Autodesk Inventor part; units mm, degrees
ref_plane "BEF_2_XY" through (32, 0, 0) normal (0, 0, 1) x (1, 0, 0)
ref_plane "BEF_2_YZ" through (32, 0, 0) normal (1, 0, 0) x (0, 1, 0)
ref_plane "BEF_2_ZX" through (32, 0, 0) normal (0, 1, 0) x (0, 0, 1)
sketch "Sketch_1" plane through (0, 0, 0) normal (0, 0, 1) x (1, 0, 0)
  line L0 (-12, -22.5) -> (98, -22.5)
  line L1 (98, -22.5) -> (98, 22.5)
  line L2 (98, 22.5) -> (-12, 22.5)
  line L3 (-12, 22.5) -> (-12, -22.5)
extrude "Extrusion1" add sketch "Sketch_1" along normal blind 200
sketch "Sketch_2" plane through (0, 0, 0) normal (0, 1, 0) x (-1, 0, 0)
  line L0 (0, 200) -> (0, 0)
  line L1 (0, 0) -> (-7, 0)
  line L2 (-7, 0) -> (-7, 4)
  line L3 (-7, 4) -> (-5.5, 4)
  line L4 (-5.5, 4) -> (-5.5, 20)
  line L5 (-5.5, 20) -> (-9, 20)
  line L6 (-9, 20) -> (-9, 200)
  line L7 (-9, 200) -> (0, 200)
  line L8 (0, 200) -> (0, 0)
revolve "Revolution1" cut sketch "Sketch_2" angle 360 about axis through (0, 0, 200) along (0, 0, 1)
pattern_linear "Rectangular Pattern1" count 2 spacing 32 along (1, 0, 0) of "Revolution1"
sketch "Sketch_8" plane through (0, 0, 200) normal (0, 0, 1) x (1, 0, 0)
  line L0 (-12, -22.5) -> (37.5, -22.5)
  line L1 (37.5, -22.5) -> (37.5, 22.5)
  line L2 (37.5, 22.5) -> (-12, 22.5)
  line L3 (-12, 22.5) -> (-12, -22.5)
extrude "Extrusion2" cut sketch "Sketch_8" against normal blind 160
sketch "Sketch_17" plane through (0, 22.5, 0) normal (0, 1, 0) x (1, 0, 0)
  arc A0 (37.5, -1.8) -> (37.5, -8.2) centre (37.5, -5) ccw
  line L0 (37.5, -8.2) -> (48.5, -8.2)
  arc A1 (48.5, -8.2) -> (48.5, -1.8) centre (48.5, -5) ccw
  line L1 (48.5, -1.8) -> (37.5, -1.8)
extrude "Extrusion3" cut sketch "Sketch_17" against normal blind 0.75
ref_plane "BEF_2_XY" through (32, 0, 0) normal (0, 0, 1) x (1, 0, 0)
ref_plane "BEF_2_YZ" through (32, 0, 0) normal (1, 0, 0) x (0, 1, 0)
ref_plane "BEF_2_ZX" through (32, 0, 0) normal (0, 1, 0) x (0, 0, 1)
ref_plane "IP_ALU_XY" through (43, 21.75, 5) normal (0, -1, 0) x (1, 0, 0)
ref_plane "IP_ALU_YZ" through (43, 21.75, 5) normal (1, 0, 0) x (0, 0, 1)
ref_plane "IP_ALU_ZX" through (43, 21.75, 5) normal (0, 0, 1) x (0, -1, 0)
ref_plane "IP_ALU_3_7_XY" through (44, 21.75, 5) normal (0, -1, 0) x (1, 0, 0)
ref_plane "IP_ALU_3_7_YZ" through (44, 21.75, 5) normal (1, 0, 0) x (0, 0, 1)
ref_plane "IP_ALU_3_7_ZX" through (44, 21.75, 5) normal (0, 0, 1) x (0, -1, 0)
ref_plane "IP_ALU_5_XY" through (44, 21.75, 5) normal (0, -1, 0) x (1, 0, 0)
ref_plane "IP_ALU_5_YZ" through (44, 21.75, 5) normal (1, 0, 0) x (0, 0, 1)
ref_plane "IP_ALU_5_ZX" through (44, 21.75, 5) normal (0, 0, 1) x (0, -1, 0)
ref_plane "IP_GR_XY" through (0, 0, 0) normal (0, 0, 1) x (1, 0, 0)
ref_plane "IP_GR_YZ" through (0, 0, 0) normal (1, 0, 0) x (0, 1, 0)
ref_plane "IP_GR_ZX" through (0, 0, 0) normal (0, 1, 0) x (0, 0, 1)
ref_plane "IP_SCH_1_XY" through (0, 0, 20) normal (0, 0, 1) x (1, 0, 0)
ref_plane "IP_SCH_1_YZ" through (0, 0, 20) normal (1, 0, 0) x (0, 1, 0)
ref_plane "IP_SCH_1_ZX" through (0, 0, 20) normal (0, 1, 0) x (0, 0, 1)
ref_plane "IP_SCH_2_XY" through (32, 0, 20) normal (0, 0, 1) x (1, 0, 0)
ref_plane "IP_SCH_2_YZ" through (32, 0, 20) normal (1, 0, 0) x (0, 1, 0)
ref_plane "IP_SCH_2_ZX" through (32, 0, 20) normal (0, 1, 0) x (0, 0, 1)
properties part number "FGR AL-2-PGN-plus-P 160,PGN-plus-P 160-2-AS-P81110452001216049.51650000000000000000Aluminium6.5"
Design review of the part built by this model. Coordinates are the model's own, in mm. A direction names the side the tool comes from. Give positions to 0.01 mm unless a question says otherwise; leave off trailing zeros. Loops run counter-clockwise (first coordinate to the right, second up) from the corner with the lowest first, then second, coordinate; pieces in that order, holes last. Notation, with made-up numbers: (-1.5, 87.5) -> (55.5, 87.5) arc R22 cw to (55.5, 114.5) -> close; hole circle Ø3 at (29, 14.25). An arc over 180 degrees is marked (long way). One line per item, written item: value.
Q1. We need section D-D on z = 85. Give the boundary of the cut face in (x, y), and give its area (3 significant figures).
Numbers:
outline: (37.5, -22.5) -> (98, -22.5) -> (98, 22.5) -> (37.5, 22.5) -> (37.5, 7.12) arc R9 cw to (37.5, -7.12) -> close
area: 2,690 mm^2
Q2. For pin 1 Ø22.5 at (x, y) = (15, -10) entering from +Z; pin 2 Ø10 at (y, z) = (7, 117) entering from -X; pin 3 Ø12.5 at (x, y) = (32, 0) entering from -Z, all flat-tipped, find the tip position at first contact; note any pin that passes through.
Numbers:
pin 1: stops at z = 40
pin 2: stops at x = 37.5
pin 3: stops at z = 4
Q3. We need section A-A on x = 32. Give the boundary of the cut face in (y, z), and give its area (3 significant figures).
Numbers:
outline: (-22.5, 0) -> (-7, 0) -> (-7, 4) -> (-5.5, 4) -> (-5.5, 20) -> (-9, 20) -> (-9, 40) -> (-22.5, 40) -> close; (5.5, 4) -> (7, 4) -> (7, 0) -> (22.5, 0) -> (22.5, 40) -> (9, 40) -> (9, 20) -> (5.5, 20) -> close
area: 1,210 mm^2
Q4. Machinability: for faces 1 (the flat face through (28, -4, 4)), 2 (the flat face through (37.5, 15, 121)), 3 (the flat face through (-4, -4, 20)), which of the approach directions +Z, -Z, +X, -X, +Y, -Y give a long, thin tool a straight path to every point of the face, cutting with its end or side? Answer none if there is none.
Numbers:
face 1: -Z
face 2: +Z, -X, +Y, -Y
face 3: +Z
Q5. For L1, parallel to Y at x = 0, z = 1; L2, parallel to Y at x = 0, z = 27.5; L3, parallel to X at y = -2, z = 13.5, list the stretches that pass through material, from the lowest coordinate up.
Numbers:
L1: y = -22.5 to -7, 7 to 22.5
L2: y = -22.5 to -9, 9 to 22.5
L3: x = -12 to -5.12, 5.12 to 26.88, 37.12 to 98
Q6. We need section C-C on z = 37. Give the boundary of the cut face in (x, y), and give its area (3 significant figures).
Numbers:
outline: (-12, -22.5) -> (98, -22.5) -> (98, 22.5) -> (-12, 22.5) -> close; hole circle Ø18 at (0, 0); hole circle Ø18 at (32, 0)
area: 4,440 mm^2
Q7. Draft analysis for pull direction Y (two halves, no side actions). For faces 4 (the flat face through (12, 0, 40)), 5 (the flat face through (43, 21.75, 5)), 6 (the flat face through (-4, -4, 4)), state which applies: pulls with the +Y half, pulls with the -Y half, needs draft (parallel to the pull), parting line crosses it, or undercut.
Numbers:
face 4: needs draft
face 5: pulls with the +Y half
face 6: undercut
Q8. We need section B-B on y = 0. Give the boundary of the cut face in (x, z).
Numbers:
outline: (-12, 0) -> (-7, 0) -> (-7, 4) -> (-5.5, 4) -> (-5.5, 20) -> (-9, 20) -> (-9, 40) -> (-12, 40) -> close; (5.5, 4) -> (7, 4) -> (7, 0) -> (25, 0) -> (25, 4) -> (26.5, 4) -> (26.5, 20) -> (23, 20) -> (23, 40) -> (9, 40) -> (9, 20) -> (5.5, 20) -> close; (37.5, 4) -> (39, 4) -> (39, 0) -> (98, 0) -> (98, 200) -> (41, 200) -> (41, 20) -> (37.5, 20) -> close
